from build123d import *

# Parameters (mm, degrees)
SKETCH_W      = 152
SKETCH_H      = 150
SKETCH_R      = 2.5
SKETCH_R_2    = 2.625
PAD_DEPTH     = 6
SKETCH001_W   = 152
SKETCH001_H   = 41
SKETCH001_R   = 8
SKETCH001_R_2 = 2.125
PAD001_DEPTH  = 6


with BuildPart() as part:
    # Sketch → Pad (new body)
    with BuildSketch(Plane.XY):
        with Locations((0, -5)):
            Rectangle(SKETCH_W, SKETCH_H)
        with Locations((-19, 55)):
            Circle(SKETCH_R, mode=Mode.SUBTRACT)
        with Locations((17, 55)):
            Circle(SKETCH_R, mode=Mode.SUBTRACT)
        with Locations((-19, -55)):
            Circle(SKETCH_R, mode=Mode.SUBTRACT)
        with Locations((17, -55)):
            Circle(SKETCH_R, mode=Mode.SUBTRACT)
        with Locations((-70, 65)):
            Circle(SKETCH_R_2, mode=Mode.SUBTRACT)
        with Locations((-40, 65)):
            Circle(SKETCH_R_2, mode=Mode.SUBTRACT)
        with Locations((-70, 39)):
            Circle(SKETCH_R_2, mode=Mode.SUBTRACT)
        with Locations((-40, 39)):
            Circle(SKETCH_R_2, mode=Mode.SUBTRACT)
        with Locations((-70, -39)):
            Circle(SKETCH_R_2, mode=Mode.SUBTRACT)
        with Locations((-40, -39)):
            Circle(SKETCH_R_2, mode=Mode.SUBTRACT)
        with Locations((-70, -65)):
            Circle(SKETCH_R_2, mode=Mode.SUBTRACT)
        with Locations((-40, -65)):
            Circle(SKETCH_R_2, mode=Mode.SUBTRACT)
        with Locations((40, 65)):
            Circle(SKETCH_R_2, mode=Mode.SUBTRACT)
        with Locations((70, 65)):
            Circle(SKETCH_R_2, mode=Mode.SUBTRACT)
        with Locations((40, 39)):
            Circle(SKETCH_R_2, mode=Mode.SUBTRACT)
        with Locations((40, -39)):
            Circle(SKETCH_R_2, mode=Mode.SUBTRACT)
        with Locations((40, -65)):
            Circle(SKETCH_R_2, mode=Mode.SUBTRACT)
        with Locations((70, -39)):
            Circle(SKETCH_R_2, mode=Mode.SUBTRACT)
        with Locations((70, -65)):
            Circle(SKETCH_R_2, mode=Mode.SUBTRACT)
        with Locations((0, 23)):
            Circle(SKETCH_R, mode=Mode.SUBTRACT)
        with Locations((15, 23)):
            Circle(SKETCH_R, mode=Mode.SUBTRACT)
        with Locations((0, -23)):
            Circle(SKETCH_R, mode=Mode.SUBTRACT)
        with Locations((15, -23)):
            Circle(SKETCH_R, mode=Mode.SUBTRACT)
        with Locations((70, 39)):
            Circle(SKETCH_R_2, mode=Mode.SUBTRACT)
    extrude(amount=PAD_DEPTH)

    # Sketch001 → Pad001 (new body)
    with BuildSketch(Plane.XZ.offset(80)):
        with Locations((0, -14.5)):
            Rectangle(SKETCH001_W, SKETCH001_H)
        with Locations((0, -16)):
            Circle(SKETCH001_R, mode=Mode.SUBTRACT)
        with Locations((-11.313708, -4.686292)):
            Circle(SKETCH001_R_2, mode=Mode.SUBTRACT)
        with Locations((-16, -16)):
            Circle(SKETCH001_R_2, mode=Mode.SUBTRACT)
        with Locations((11.313708, -4.686292)):
            Circle(SKETCH001_R_2, mode=Mode.SUBTRACT)
        with Locations((-11.313708, -27.313708)):
            Circle(SKETCH001_R_2, mode=Mode.SUBTRACT)
        with Locations((11.313708, -27.313708)):
            Circle(SKETCH001_R_2, mode=Mode.SUBTRACT)
        with Locations((16, -16)):
            Circle(SKETCH001_R_2, mode=Mode.SUBTRACT)
        with Locations((-55, -15)):
            Circle(SKETCH001_R, mode=Mode.SUBTRACT)
        with Locations((55, -15)):
            Circle(SKETCH001_R, mode=Mode.SUBTRACT)
    extrude(amount=-PAD001_DEPTH)


solid = part.part
Geometry: final body of the model. Coordinates: model frame, mm. A direction names the side the tool comes from. Give positions to 0.01 mm unless a question says otherwise; leave off trailing zeros. Write each loop counter-clockwise with the first axis right and the second up, starting at its lowest first coordinate (ties: lowest second). Pieces come first, ordered by that corner, then holes.
(1) Cut plane D-D, the plane x = 0. Return loops of the section in (y, z), then the cut area to 3 significant figures.
(2) Cut plane C-C, the plane y = 65. Return loops of the section in (x, z) (3 decimals).
(3) Cut plane B-B, the plane x = -70. Return loops of the section in (y, z) (3 decimals).
(4) Ray query, line 1 (Y direction, x = 40, z = 2) (3 decimals); line 2 (Y direction, x = -19, z = 1.85); line 3 (Y direction, x = 63, z = -29). Return the intervals inside material, ascending.
(5) Access query for faces 1 (the cylindrical face through (48.651, -77.042, -19.868)), 2 (the flat face through (-1, -1, 0)). Directions: +Z, -Z, +X, -X, +Y, -Y. A direction counts if a zero-diameter tool reaches every point of the face in a straight line with its end or side. Return the directions, or none.
(6) Cut plane A-A, the plane y = 23. Return loops of the section in (x, z), then the cut area to 3 significant figures.
(7) First-contact query: P1, Ø2, axis at x = -44.5, y = 54, coming from the -Z side; P2, Ø1.5, axis at x = 13.5, z = -7.5, coming from the +Y side. Flat tips, straight axial feed; report the tip coordinate or a pass-through.
(8) Mould query, pull axis X, two halves, no side actions, for faces 3 (the cylindrical face through (-67.575, 63.995, 2.958)), 4 (the flat face through (-1, 70, 3)), 5 (the flat face through (76, -16, 2)). Classes: released by +X, released by -X, zero draft, split by the parting line, or undercut.
Values follow:
1. outline: (-80, -35) - (-74, -35) - (-74, -24) - (-80, -24) - close; (-80, -8) - (-74, -8) - (-74, 0) - (-25.5, 0) - (-25.5, 6) - (-80, 6) - close; (-20.5, 0) - (20.5, 0) - (20.5, 6) - (-20.5, 6) - close; (25.5, 0) - (70, 0) - (70, 6) - (25.5, 6) - close
1. area: 954 mm2
2. outline: (-76, 0) - (-72.625, 0) - (-72.625, 6) - (-76, 6) - close; (-67.375, 0) - (-42.625, 0) - (-42.625, 6) - (-67.375, 6) - close; (-37.375, 0) - (37.375, 0) - (37.375, 6) - (-37.375, 6) - close; (42.625, 0) - (67.375, 0) - (67.375, 6) - (42.625, 6) - close; (72.625, 0) - (76, 0) - (76, 6) - (72.625, 6) - close
3. outline: (-80, -35) - (-74, -35) - (-74, 0) - (-67.625, 0) - (-67.625, 6) - (-80, 6) - close; (-62.375, 0) - (-41.625, 0) - (-41.625, 6) - (-62.375, 6) - close; (-36.375, 0) - (36.375, 0) - (36.375, 6) - (-36.375, 6) - close; (41.625, 0) - (62.375, 0) - (62.375, 6) - (41.625, 6) - close; (67.625, 0) - (70, 0) - (70, 6) - (67.625, 6) - close
4. line 1: y = -80 to -67.625, -62.375 to -41.625, -36.375 to 36.375, 41.625 to 62.375, 67.625 to 70
4. line 2: y = -80 to -57.5, -52.5 to 52.5, 57.5 to 70
4. line 3: y = -80 to -74
5. face 1: +Y, -Y
5. face 2: -Z, +X, -X, +Y
6. outline: (-76, 0) - (-2.5, 0) - (-2.5, 6) - (-76, 6) - close; (2.5, 0) - (12.5, 0) - (12.5, 6) - (2.5, 6) - close; (17.5, 0) - (76, 0) - (76, 6) - (17.5, 6) - close
6. area: 852 mm2
7. P1: stops at z = 0
7. P2: stops at y = -74
8. face 3: undercut
8. face 4: zero draft
8. face 5: released by +X
